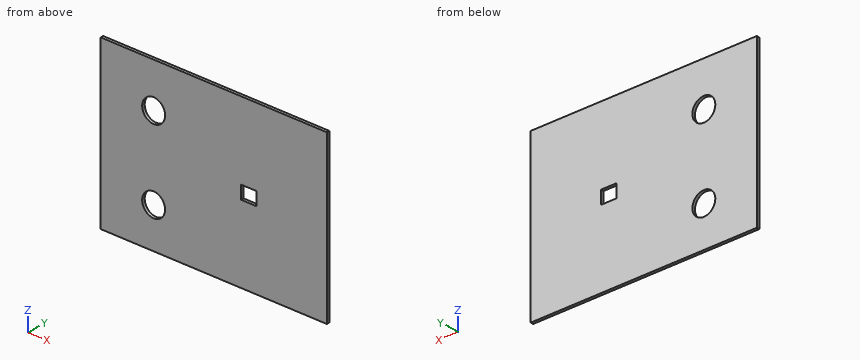
from build123d import *

# Parameters (mm, degrees)
F0_W     = 1003.3
F0_H     = 723.9
F1_DEPTH = 12.7
F2_W     = 69.85
F2_H     = 57.15
F3_DEPTH = 12.701
F4_R     = 50.8
F5_DEPTH = 12.701


with BuildPart() as f1:
    # F0 (on Front) → F1 (new body)
    with BuildSketch(Plane.XZ):
        with Locations((-501.65, 0)):
            Rectangle(F0_W, F0_H)
    extrude(amount=F1_DEPTH)

    # F2 (on Front) → F3 (cut, through all)
    with BuildSketch(Plane.XZ):
        with Locations((-346.075, 0)):
            Rectangle(F2_W, F2_H)
    extrude(amount=F3_DEPTH, mode=Mode.SUBTRACT)

    # F4 (on Front) → F5 (cut, through all)
    with BuildSketch(Plane.XZ):
        with Locations((-768.35, 169.221888)):
            Circle(F4_R)
        with Locations((-768.35, -186.378112)):
            Circle(F4_R)
    extrude(amount=F5_DEPTH, mode=Mode.SUBTRACT)


solid = f1.part
Input: part model. Units: mm. Frame: model coordinates. Coordinates: 2 decimals unless noted, no trailing zeros. Loops run counter-clockwise (first coordinate to the right, second up) from the corner with the lowest first, then second, coordinate; pieces in that order, holes last.
(1) Section C-C on y = -10.5. Return the cut outline in (x, z) (3 decimals).
(2) Material intervals for probe 1 along Z at (x, y) = (-771, -9); probe 2 along Z at (x, y) = (-768.35, -4.5); probe 3 along Z at (x, y) = (-377.5, -6.25) (3 decimals), sorted ascending.
(3) Section B-B on x = -768.35. Return the cut outline in (y, z), then the cut area to 3 significant figures.
(4) Section A-A on z = -12. Return the cut outline in (x, y), then the cut area to 3 significant figures.
Data:
1. outline: (-1003.3, -361.95) - (0, -361.95) - (0, 361.95) - (-1003.3, 361.95) - close; hole circle Ø101.6 at (-768.35, -186.378); hole circle Ø101.6 at (-768.35, 169.222); hole (-381, -28.575) - (-311.15, -28.575) - (-311.15, 28.575) - (-381, 28.575) - close
2. probe 1: z = -361.95 to -237.11, -135.65 to 118.49, 219.95 to 361.95
2. probe 2: z = -361.95 to -237.18, -135.58 to 118.42, 220.02 to 361.95
2. probe 3: z = -361.95 to -28.575, 28.575 to 361.95
3. outline: (-12.7, -361.95) - (0, -361.95) - (0, -237.18) - (-12.7, -237.18) - close; (-12.7, -135.58) - (0, -135.58) - (0, 118.42) - (-12.7, 118.42) - close; (-12.7, 220.02) - (0, 220.02) - (0, 361.95) - (-12.7, 361.95) - close
3. area: 6,610 mm2
4. outline: (-1003.3, -12.7) - (-381, -12.7) - (-381, 0) - (-1003.3, 0) - close; (-311.15, -12.7) - (0, -12.7) - (0, 0) - (-311.15, 0) - close
4. area: 11,900 mm2
